```python
from build123d import *

# Parameters (mm, degrees)
SKETCH1_R           = 1
SKETCH1_R_2         = 1.6
BOSS_EXTRUDE1_DEPTH = 3
SKETCH7_R           = 0.75
BOSS_EXTRUDE4_DEPTH = 0.05
SKETCH8_R           = 2.5
CUT_EXTRUDE7_DEPTH  = 10


with BuildPart() as part:
    # Sketch1 → Boss-Extrude1 (new body)
    with BuildSketch(Plane(origin=(0, 0, 0), x_dir=(1, 0, 0), z_dir=(0, 1, 0))):
        Polygon((43.076410298, 50.123925917), (42.618597625, 48.402115535), (19.4637773, 25.158118275), (-19.4637773, 25.158118275), (-42.618597625, 48.402115535), (-45.64603124, 59.788140743), (-55.300297258, 62.394891143), (-62.384942335, 55.337426715), (-59.815321393, 45.673211889), (-50.185022628, 43.072932893), (-35, 26.288270568), (-34.873, 0), (-35, -26.288270568), (-50.185022628, -43.072932893), (-59.815321393, -45.673211889), (-62.384942335, -55.337426715), (-55.300297258, -62.394891143), (-45.64603124, -59.788140743), (-42.618597625, -48.402115535), (-19.4637773, -25.158118275), (19.4637773, -25.158118275), (42.618597625, -48.402115535), (45.64603124, -59.788140743), (55.300297258, -62.394891143), (62.384942335, -55.337426715), (59.815321393, -45.673211889), (50.185022628, -43.072932893), (35, -26.288270568), (34.873, 0), (35, 26.288270568), (50.185022628, 43.072932893), (59.815321393, 45.673211889), (62.384942335, 55.337426715), (55.300297258, 62.394891143), (45.64603124, 59.788140743), align=None)
        with Locations(Location((-52.730676316, -57.230676316, 0), (0, 0, 270))):
            Circle(SKETCH1_R, mode=Mode.SUBTRACT)
        with Locations(Location((-57.230676316, -52.730676316, 0), (0, 0, 270))):
            Circle(SKETCH1_R, mode=Mode.SUBTRACT)
        with Locations(Location((-48.230676316, -52.730676316, 0), (0, 0, 270))):
            Circle(SKETCH1_R, mode=Mode.SUBTRACT)
        with Locations(Location((-52.730676316, -48.230676316, 0), (0, 0, 270))):
            Circle(SKETCH1_R, mode=Mode.SUBTRACT)
        with Locations(Location((-30, -17, 0), (0, 0, 270))):
            Circle(SKETCH1_R, mode=Mode.SUBTRACT)
        with Locations(Location((-15.25, -15.25, 0), (0, 0, 270))):
            Circle(SKETCH1_R_2, mode=Mode.SUBTRACT)
        with Locations(Location((52.730676316, -57.230676316, 0), (0, 0, 270))):
            Circle(SKETCH1_R, mode=Mode.SUBTRACT)
        with Locations(Location((48.230676316, -52.730676316, 0), (0, 0, 270))):
            Circle(SKETCH1_R, mode=Mode.SUBTRACT)
        with Locations(Location((52.730676316, -48.230676316, 0), (0, 0, 270))):
            Circle(SKETCH1_R, mode=Mode.SUBTRACT)
        with Locations(Location((57.230676316, -52.730676316, 0), (0, 0, 270))):
            Circle(SKETCH1_R, mode=Mode.SUBTRACT)
        with Locations(Location((30, -17, 0), (0, 0, 270))):
            Circle(SKETCH1_R, mode=Mode.SUBTRACT)
        with Locations(Location((15.25, -15.25, 0), (0, 0, 270))):
            Circle(SKETCH1_R_2, mode=Mode.SUBTRACT)
        with Locations(Location((-15.25, 15.25, 0), (0, 0, 270))):
            Circle(SKETCH1_R_2, mode=Mode.SUBTRACT)
        with Locations(Location((-30, 17, 0), (0, 0, 270))):
            Circle(SKETCH1_R, mode=Mode.SUBTRACT)
        with Locations(Location((-57.230676316, 52.730676316, 0), (0, 0, 270))):
            Circle(SKETCH1_R, mode=Mode.SUBTRACT)
        with Locations(Location((-52.730676316, 48.230676316, 0), (0, 0, 270))):
            Circle(SKETCH1_R, mode=Mode.SUBTRACT)
        with Locations(Location((-48.230676316, 52.730676316, 0), (0, 0, 270))):
            Circle(SKETCH1_R, mode=Mode.SUBTRACT)
        with Locations(Location((-52.730676316, 57.230676316, 0), (0, 0, 270))):
            Circle(SKETCH1_R, mode=Mode.SUBTRACT)
        with Locations(Location((15.25, 15.25, 0), (0, 0, 270))):
            Circle(SKETCH1_R_2, mode=Mode.SUBTRACT)
        with Locations(Location((30, 17, 0), (0, 0, 270))):
            Circle(SKETCH1_R, mode=Mode.SUBTRACT)
        with Locations(Location((52.730676316, 48.230676316, 0), (0, 0, 270))):
            Circle(SKETCH1_R, mode=Mode.SUBTRACT)
        with Locations(Location((48.230676316, 52.730676316, 0), (0, 0, 270))):
            Circle(SKETCH1_R, mode=Mode.SUBTRACT)
        with Locations(Location((57.230676316, 52.730676316, 0), (0, 0, 270))):
            Circle(SKETCH1_R, mode=Mode.SUBTRACT)
        with Locations(Location((52.730676316, 57.230676316, 0), (0, 0, 270))):
            Circle(SKETCH1_R, mode=Mode.SUBTRACT)
    extrude(amount=BOSS_EXTRUDE1_DEPTH)

    # Sketch7 → Boss-Extrude4 (add)
    with BuildSketch(Plane(origin=(0, 3, 0), x_dir=(1, 0, 0), z_dir=(0, 1, 0))):
        with Locations(Location((-52.730676316, -52.730676316, 0), (0, 0, 270))):
            Circle(SKETCH7_R)
        with Locations(Location((-52.730676316, 52.730676316, 0), (0, 0, 90))):
            Circle(SKETCH7_R)
        with Locations(Location((52.730676316, 52.730676316, 0), (0, 0, 270))):
            Circle(SKETCH7_R)
        with Locations(Location((52.730676316, -52.730676316, 0), (0, 0, 90))):
            Circle(SKETCH7_R)
    extrude(amount=BOSS_EXTRUDE4_DEPTH)

    # Sketch8 → Cut-Extrude7 (cut)
    with BuildSketch(Plane(origin=(0, 3, 0), x_dir=(1, 0, 0), z_dir=(0, 1, 0))):
        with Locations(Location((-52.730676316, -52.730676316, 0), (0, 0, 270))):
            Circle(SKETCH8_R)
        with Locations(Location((52.769323684, -52.730676316, 0), (0, 0, 270))):
            Circle(SKETCH8_R)
        with Locations(Location((52.769323684, 52.769323684, 0), (0, 0, 270))):
            Circle(SKETCH8_R)
        with Locations(Location((-52.730676316, 52.769323684, 0), (0, 0, 270))):
            Circle(SKETCH8_R)
    extrude(amount=-CUT_EXTRUDE7_DEPTH, mode=Mode.SUBTRACT)


with BuildPart() as body_2:
    # of the pieces the cut leaves, the one that is kept (cut_extrude7_keep)
    add(part.part.solids().sort_by_distance((-19.4637773, 0, 25.158118275))[0])


solid = body_2.part
```
Geometry: final body of the model. Coordinates: model frame, mm. A direction names the side the tool comes from. Round coordinates to 2 decimals unless told otherwise and drop trailing zeros. Write each loop counter-clockwise with the first axis right and the second up, starting at its lowest first coordinate (ties: lowest second). Pieces come first, ordered by that corner, then holes. Notation, with made-up numbers: (-36, 49.5) -> (17, 49.5) arc R25 cw to (17, 85.5) -> close; hole circle Ø10 at (17.25, 31.25). An arc over 180 degrees is marked (long way). Use CSV: the item, a comma, the result in double quotes. Start each with the question number.
Q1. Line query: L1, parallel to X at y = 1.7, z = 17; L2, parallel to X at y = 2.1, z = -51.5; L3, parallel to X at y = 2.3, z = 48.5. Output: solid intervals per line, ascending.
Q2. Section D-D (z = 34.5). Return loops of the section in (x, y), plus the area to 3 significant figures.
Q3. Section A-A (x = 15.25). Return loops of the section in (y, z).
Q4. Section B-B (z = -37). Return loops of the section in (x, y), plus the area to 3 significant figures.
Q5. Section C-C (y = 2). Give the number of separate pieces and of enclosed holes in the cut face, plus the area to 3 significant figures.
Q6. Pull-direction query (X, two-part tool) for faces 4 (the face through (51.81, 1.52, -50.46)), 5 (the face through (-58.89, 1.48, 58.82)), 6 (the face through (0, 3, 0)), 7 (the face through (-50.406, 1.479, -61.073)); classes: pulls with the +X half, pulls with the -X half, needs draft (parallel to the pull), parting line crosses it, or undercut.
Q7. Reachability of faces 1 (the face through (42.486, 1.479, -34.563)), 2 (the face through (50.5, 1.5, -61.1)), 3 (the face through (-61.118, 1.479, -50.573)) from +Z, -Z, +X, -X, +Y, -Y: full face, straight path, thin tool, end or side. Return the list, or none.
Result sheet:
1,L1,"-34.96 to -31, -29 to 29, 31 to 34.96"
1,L2,"-61.36 to -54.88, -50.58 to -43.44, 43.44 to 50.62, 54.92 to 61.36"
1,L3,"-60.57 to -53.69, -51.77 to -42.64, 42.64 to 51.77, 53.69 to 60.57"
2,outline,"(-42.43, 0) -> (-28.77, 0) -> (-28.77, 3) -> (-42.43, 3) -> close; (28.77, 0) -> (42.43, 0) -> (42.43, 3) -> (28.77, 3) -> close"
2,area,"82.0 mm²"
3,outline,"(0, -25.16) -> (3, -25.16) -> (3, -16.85) -> (0, -16.85) -> close; (0, -13.65) -> (3, -13.65) -> (3, 13.65) -> (0, 13.65) -> close; (0, 16.85) -> (3, 16.85) -> (3, 25.16) -> (0, 25.16) -> close"
4,outline,"(-44.69, 0) -> (-31.26, 0) -> (-31.26, 3) -> (-44.69, 3) -> close; (31.26, 0) -> (44.69, 0) -> (44.69, 3) -> (31.26, 3) -> close"
4,area,"80.6 mm²"
5,separate pieces,"1"
5,enclosed holes,"28"
5,area,"5,530 mm²"
6,face 4,"undercut"
6,face 5,"pulls with the -X half"
6,face 6,"needs draft"
6,face 7,"undercut"
7,face 1,"+X, +Y, -Y"
7,face 2,"-Z, +Y, -Y"
7,face 3,"-X, +Y, -Y"
